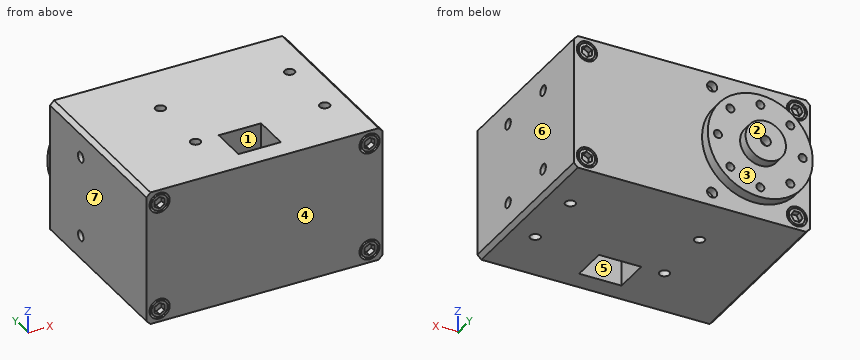
from build123d import *

# Parameters (mm, degrees)
BOSS_EXTRUDE1_DEPTH = 44
SKETCH2_R           = 13
SKETCH2_R_2         = 1
BOSS_EXTRUDE2_DEPTH = 2.65
SKETCH3_R           = 5
SKETCH3_R_2         = 1.25
BOSS_EXTRUDE3_DEPTH = 2.5
SKETCH4_R           = 2.5
SKETCH4_R_2         = 1.25
CUT_EXTRUDE1_DEPTH  = 2
SKETCH5_R           = 1.25
CUT_EXTRUDE2_DEPTH  = 2
SKETCH6_R           = 13
SKETCH6_R_2         = 1.25
BOSS_EXTRUDE4_DEPTH = 2.5
SKETCH7_R           = 2.5
CUT_EXTRUDE3_DEPTH  = 2.5
SKETCH8_R           = 1.25
CUT_EXTRUDE4_DEPTH  = 2.5
SKETCH9_R           = 1.25
CUT_EXTRUDE5_DEPTH  = 2.5
SKETCH10_W          = 10.5
SKETCH10_H          = 9
CUT_EXTRUDE6_DEPTH  = 7
SKETCH11_R          = 13
CUT_EXTRUDE7_DEPTH  = 2.5
SKETCH13_R          = 2
BOSS_EXTRUDE5_DEPTH = 2
CUT_EXTRUDE8_DEPTH  = 1.5
SKETCH15_R          = 2
BOSS_EXTRUDE6_DEPTH = 2.5
CUT_EXTRUDE9_DEPTH  = 1.5


with BuildPart() as part:
    # Sketch1 → Boss-Extrude1 (new body)
    with BuildSketch(Plane(origin=(0, 0, 0), x_dir=(1, 0, 0), z_dir=(0, 1, 0))):
        Polygon((-29.25, -15.75), (-28.25, -16.75), (28.25, -16.75), (29.25, -15.75), (29.25, 15.75), (28.25, 16.75), (-28.25, 16.75), (-29.25, 15.75), align=None)
    extrude(amount=BOSS_EXTRUDE1_DEPTH)

    # Sketch2 → Boss-Extrude2 (add)
    with BuildSketch(Plane(origin=(0, 44, 0), x_dir=(1, 0, 0), z_dir=(0, 1, 0))):
        with Locations((-15.5, 0)):
            Circle(SKETCH2_R)
        with Locations((-15.5, 10.5)):
            Circle(SKETCH2_R_2, mode=Mode.SUBTRACT)
        with Locations((-8.075378798, 7.424621202)):
            Circle(SKETCH2_R_2, mode=Mode.SUBTRACT)
        with Locations((-5, 0)):
            Circle(SKETCH2_R_2, mode=Mode.SUBTRACT)
        with Locations((-8.075378798, -7.424621202)):
            Circle(SKETCH2_R_2, mode=Mode.SUBTRACT)
        with Locations((-15.5, -10.5)):
            Circle(SKETCH2_R_2, mode=Mode.SUBTRACT)
        with Locations((-22.924621202, -7.424621202)):
            Circle(SKETCH2_R_2, mode=Mode.SUBTRACT)
        with Locations((-26, 0)):
            Circle(SKETCH2_R_2, mode=Mode.SUBTRACT)
        with Locations((-22.924621202, 7.424621202)):
            Circle(SKETCH2_R_2, mode=Mode.SUBTRACT)
    extrude(amount=BOSS_EXTRUDE2_DEPTH)

    # Sketch3 → Boss-Extrude3 (add)
    with BuildSketch(Plane(origin=(0, 46.65, 0), x_dir=(1, 0, 0), z_dir=(0, 1, 0))):
        with Locations((-15.5, 0)):
            Circle(SKETCH3_R)
        with Locations((-15.5, 0)):
            Circle(SKETCH3_R_2, mode=Mode.SUBTRACT)
    extrude(amount=BOSS_EXTRUDE3_DEPTH)

    # Sketch4 → Cut-Extrude1 (cut)
    with BuildSketch(Plane(origin=(0, 44, 0), x_dir=(1, 0, 0), z_dir=(0, 1, 0))):
        with Locations((-26, 13.5)):
            Circle(SKETCH4_R)
        with Locations((-26, -13.5)):
            Circle(SKETCH4_R)
        with Locations((26, -13.5)):
            Circle(SKETCH4_R)
        with Locations((26, 13.5)):
            Circle(SKETCH4_R)
        with Locations((-5, 13.5)):
            Circle(SKETCH4_R_2)
        with Locations((-5, -13.5)):
            Circle(SKETCH4_R_2)
    extrude(amount=-CUT_EXTRUDE1_DEPTH, mode=Mode.SUBTRACT)

    # Sketch5 → Cut-Extrude2 (cut)
    with BuildSketch(Plane.XY.offset(16.75)):
        with Locations((-9.5, 30)):
            Circle(SKETCH5_R)
        with Locations((-9.5, 14)):
            Circle(SKETCH5_R)
        with Locations((22.5, 30)):
            Circle(SKETCH5_R)
        with Locations((22.5, 14)):
            Circle(SKETCH5_R)
    cut_extrude2 = extrude(amount=-CUT_EXTRUDE2_DEPTH, mode=Mode.SUBTRACT)

    # Sketch6 → Boss-Extrude4 (add)
    with BuildSketch(Plane.XZ):
        with Locations((-15.5, 0)):
            Circle(SKETCH6_R)
        with Locations((-5, 0)):
            Circle(SKETCH6_R_2, mode=Mode.SUBTRACT)
        with Locations((-8.075378798, -7.424621202)):
            Circle(SKETCH6_R_2, mode=Mode.SUBTRACT)
        with Locations((-15.5, -10.5)):
            Circle(SKETCH6_R_2, mode=Mode.SUBTRACT)
        with Locations((-22.924621202, -7.424621202)):
            Circle(SKETCH6_R_2, mode=Mode.SUBTRACT)
        with Locations((-26, 0)):
            Circle(SKETCH6_R_2, mode=Mode.SUBTRACT)
        with Locations((-22.924621202, 7.424621202)):
            Circle(SKETCH6_R_2, mode=Mode.SUBTRACT)
        with Locations((-15.5, 10.5)):
            Circle(SKETCH6_R_2, mode=Mode.SUBTRACT)
        with Locations((-8.075378798, 7.424621202)):
            Circle(SKETCH6_R_2, mode=Mode.SUBTRACT)
    extrude(amount=BOSS_EXTRUDE4_DEPTH)

    # Sketch7 → Cut-Extrude3 (cut)
    with BuildSketch(Plane.XZ):
        with Locations((-26, 13.5)):
            Circle(SKETCH7_R)
        with Locations((-26, -13.5)):
            Circle(SKETCH7_R)
        with Locations((26, -13.5)):
            Circle(SKETCH7_R)
        with Locations((26, 13.5)):
            Circle(SKETCH7_R)
    extrude(amount=-CUT_EXTRUDE3_DEPTH, mode=Mode.SUBTRACT)

    # Sketch8 → Cut-Extrude4 (cut)
    with BuildSketch(Plane(origin=(29.25, 0, 0), x_dir=(0, 0, -1), z_dir=(1, 0, 0))):
        with Locations((-10, 14)):
            Circle(SKETCH8_R)
        with Locations((10, 14)):
            Circle(SKETCH8_R)
        with Locations((10, 30)):
            Circle(SKETCH8_R)
        with Locations((-10, 30)):
            Circle(SKETCH8_R)
    extrude(amount=-CUT_EXTRUDE4_DEPTH, mode=Mode.SUBTRACT)

    # Sketch9 → Cut-Extrude5 (cut)
    with BuildSketch(Plane.ZY.offset(29.25)):
        with Locations((-10, 30)):
            Circle(SKETCH9_R)
        with Locations((10, 30)):
            Circle(SKETCH9_R)
    extrude(amount=-CUT_EXTRUDE5_DEPTH, mode=Mode.SUBTRACT)

    # Sketch10 → Cut-Extrude6 (cut)
    with BuildSketch(Plane.XY.offset(16.75)):
        with Locations((1.5, 9.5)):
            Rectangle(SKETCH10_W, SKETCH10_H)
    cut_extrude6 = extrude(amount=-CUT_EXTRUDE6_DEPTH, mode=Mode.SUBTRACT)

    # Mirror1: Cut-Extrude6 across plane
    add(cut_extrude6.mirror(Plane.XY), mode=Mode.SUBTRACT)

    # Mirror2: Cut-Extrude2 across plane
    add(cut_extrude2.mirror(Plane.XY), mode=Mode.SUBTRACT)

    # Sketch11 → Cut-Extrude7 (cut)
    with BuildSketch(Plane.XZ.offset(2.5)):
        with Locations((-15.5, 0)):
            Circle(SKETCH11_R)
    extrude(amount=-CUT_EXTRUDE7_DEPTH, mode=Mode.SUBTRACT)

    # Sketch13 → Boss-Extrude5 (add)
    with BuildSketch(Plane(origin=(0, 42, 0), x_dir=(1, 0, 0), z_dir=(0, 1, 0))):
        with Locations((-26, 13.5)):
            Circle(SKETCH13_R)
        with Locations((-26, -13.5)):
            Circle(SKETCH13_R)
        with Locations((26, 13.5)):
            Circle(SKETCH13_R)
        with Locations((26, -13.5)):
            Circle(SKETCH13_R)
    extrude(amount=BOSS_EXTRUDE5_DEPTH)

    # Sketch14 → Cut-Extrude8 (cut)
    with BuildSketch(Plane(origin=(0, 44, 0), x_dir=(1, 0, 0), z_dir=(0, 1, 0))):
        Polygon((-27.443375673, 13.5), (-26.721687836, 12.25), (-25.278312164, 12.25), (-24.556624327, 13.5), (-25.278312164, 14.75), (-26.721687836, 14.75), align=None)
        Polygon((24.709537385, 14.146559797), (24.794831483, 12.705706491), (26.085294098, 12.059146694), (27.290462615, 12.853440203), (27.205168517, 14.294293509), (25.914705902, 14.940853306), align=None)
        Polygon((-26.694922261, -12.234924356), (-27.443048776, -13.469282509), (-26.748126515, -14.734358153), (-25.305077739, -14.765075644), (-24.556951224, -13.530717491), (-25.251873485, -12.265641847), align=None)
        Polygon((24.754214587, -14.228938982), (26.00838697, -14.943351306), (27.254172382, -14.214412324), (27.245785413, -12.771061018), (25.99161303, -12.056648694), (24.745827618, -12.785587676), align=None)
    extrude(amount=-CUT_EXTRUDE8_DEPTH, mode=Mode.SUBTRACT)

    # Sketch15 → Boss-Extrude6 (add)
    with BuildSketch(Plane.XZ.offset(-2.5)):
        with Locations((-26, 13.5)):
            Circle(SKETCH15_R)
        with Locations((26, 13.5)):
            Circle(SKETCH15_R)
        with Locations((-26, -13.5)):
            Circle(SKETCH15_R)
        with Locations((26, -13.5)):
            Circle(SKETCH15_R)
    extrude(amount=BOSS_EXTRUDE6_DEPTH)

    # Sketch16 → Cut-Extrude9 (cut)
    with BuildSketch(Plane.XZ):
        Polygon((-26, 12.056624327), (-24.75, 12.778312164), (-24.75, 14.221687836), (-26, 14.943375673), (-27.25, 14.221687836), (-27.25, 12.778312164), align=None)
        Polygon((26, 12.056624327), (27.25, 12.778312164), (27.25, 14.221687836), (26, 14.943375673), (24.75, 14.221687836), (24.75, 12.778312164), align=None)
        Polygon((26, -14.943375673), (27.25, -14.221687836), (27.25, -12.778312164), (26, -12.056624327), (24.75, -12.778312164), (24.75, -14.221687836), align=None)
        Polygon((-26, -14.943375673), (-24.75, -14.221687836), (-24.75, -12.778312164), (-26, -12.056624327), (-27.25, -12.778312164), (-27.25, -14.221687836), align=None)
    extrude(amount=-CUT_EXTRUDE9_DEPTH, mode=Mode.SUBTRACT)


solid = part.part
Geometry: final body of the model. Coordinates: model frame, mm. Face numbers are marked on the shaded views. A direction names the side the tool comes from. Coordinates: 2 decimals unless noted, no trailing zeros. Loops run counter-clockwise (first coordinate to the right, second up) from the corner with the lowest first, then second, coordinate; pieces in that order, holes last. Notation, with made-up numbers: M 39,-16.5 L 82,-16.5 A33 cw 82,11.5 Z; hole C -1,67.25 d5. An arc over 180 degrees is marked long. One line per item, written item: value. Start each with the question number.
1) Draft query along X for the marked faces 4, 5, 6 and 7. Return one class per face: released by +X, released by -X, zero draft, split by the parting line, or undercut.
2) Material intervals for L1, parallel to Y at x = 22.5, z = 15.45; L2, parallel to Z at x = -15.5, y = 45.1; L3, parallel to Y at x = 22, z = -15, sorted ascending. Write a range as from..to.
3) Cut plane C-C (x = -15.5). Return loops of the section in (y, z).
4) Pin query (flat end, axial travel): P1, Ø6.5, axis at x = 26, z = -13.5, coming from the +Y side; P2, Ø1.6, axis at x = -22.5, z = 7.5, coming from the +Y side; P3, Ø1.2, axis at y = 30, z = -10.5, coming from the -X side. Return the tip coordinate at first contact, or that it passes through.
5) Cut plane A-A (x = -5). Return loops of the section in (y, z).
6) Reachability of the marked faces 1, 2 and 3 from +Z, -Z, +X, -X, +Y, -Y: full face, straight path, thin tool, end or side. Return the list, or none.
7) Cut plane B-B (x = 22.5). Return loops of the section in (y, z), then the cut area to 3 significant figures.
Evaluation:
1. face 4: zero draft
1. face 5: undercut
1. face 6: released by +X
1. face 7: released by -X
2. L1: 0..12.75, 15.25..28.75, 31.25..44
2. L2: -13..-11.5, -9.5..9.5, 11.5..13
2. L3: 0..12.85, 15.15..28.85, 31.15..44
3. outline: M 0,-16.75 L 44,-16.75 L 44,-13 L 46.65,-13 L 46.65,-11.5 L 44,-11.5 L 44,-9.5 L 46.65,-9.5 L 46.65,-5 L 49.15,-5 L 49.15,-1.25 L 46.65,-1.25 L 46.65,1.25 L 49.15,1.25 L 49.15,5 L 46.65,5 L 46.65,9.5 L 44,9.5 L 44,11.5 L 46.65,11.5 L 46.65,13 L 44,13 L 44,16.75 L 0,16.75 Z
4. P1: y = 44
4. P2: y = 46.65
4. P3: x = -26.75
5. outline: M 0,-16.75 L 44,-16.75 L 44,-14.75 L 42,-14.75 L 42,-12.25 L 44,-12.25 L 44,-7.66 L 46.65,-7.66 L 46.65,-1 L 44,-1 L 44,1 L 46.65,1 L 46.65,7.66 L 44,7.66 L 44,12.25 L 42,12.25 L 42,14.75 L 44,14.75 L 44,16.75 L 0,16.75 Z
6. face 1: +Z
6. face 2: +Z, -Z, +X, -X, +Y
6. face 3: +Y
7. outline: M 0,-16.75 L 12.75,-16.75 L 12.75,-14.75 L 15.25,-14.75 L 15.25,-16.75 L 28.75,-16.75 L 28.75,-14.75 L 31.25,-14.75 L 31.25,-16.75 L 44,-16.75 L 44,16.75 L 31.25,16.75 L 31.25,14.75 L 28.75,14.75 L 28.75,16.75 L 15.25,16.75 L 15.25,14.75 L 12.75,14.75 L 12.75,16.75 L 0,16.75 Z
7. area: 1,450 mm^2
